Design review of the part built by this model. Coordinates are the model's own, in mm. A direction names the side the tool comes from. Give positions to 0.01 mm unless a question says otherwise; leave off trailing zeros. Order: outer loops, then holes, each group sorted by start corner. A loop starts at its lowest first (then second) coordinate and runs counter-clockwise, first axis right, second up.
```python
from build123d import *

# Parameters (mm, degrees)
BOSS_EXTRUDE1_DEPTH = 20
FILLET1_R           = 1
SKETCH2_R           = 9
CUT_EXTRUDE1_DEPTH  = 20
BOSS_EXTRUDE2_START = 2
BOSS_EXTRUDE2_DEPTH = 2
SKETCH4_W           = 20
SKETCH4_H           = 20
BOSS_EXTRUDE3_DEPTH = 2
FILLET2_R           = 1
SKETCH5_W           = 12.5
SKETCH5_H           = 2
CUT_EXTRUDE2_DEPTH  = 24
BOSS_EXTRUDE4_DEPTH = 80
FILLET3_R           = 1
SKETCH8_R           = 7.11392485
SKETCH8_W           = 20
SKETCH8_H           = 40
CUT_EXTRUDE3_DEPTH  = 2
SKETCH9_W           = 20
SKETCH9_H           = 2
BOSS_EXTRUDE5_DEPTH = 15
FILLET4_R           = 1
SKETCH10_R          = 2.5
CUT_EXTRUDE4_DEPTH  = 20
CUT_EXTRUDE5_DEPTH  = 1000
SKETCH12_W          = 38.052123651
SKETCH12_H          = 24.689337754
CUT_EXTRUDE6_DEPTH  = 200


with BuildPart() as part:
    # Sketch1 → Boss-Extrude1 (new body)
    with BuildSketch(Plane(origin=(0, 0, 0), x_dir=(1, 0, 0), z_dir=(0, 1, 0))):
        Polygon((-2.291666667, 11.041666667), (-22.291666667, 11.041666667), (-22.291666667, -8.958333333), (-2.291666667, -8.958333333), (-2.291666667, -6.958333333), (-20.291666667, -6.958333333), (-20.291666667, 9.041666667), (-2.291666667, 9.041666667), align=None)
    extrude(amount=BOSS_EXTRUDE1_DEPTH)

    # Fillet1
    fillet1_edges = [part.edges().sort_by_distance(p)[0] for p in [
        (-22.291666667, 10, 8.958333333),
        (-22.291666667, 10, -11.041666667),
    ]]
    fillet(fillet1_edges, radius=FILLET1_R)

    # Sketch2 → Cut-Extrude1 (cut)
    with BuildSketch(Plane.XY.offset(8.958333333)):
        with Locations(Location((-12.291666667, 10, 0), (0, 0, 180))):
            Circle(SKETCH2_R)
    extrude(amount=-CUT_EXTRUDE1_DEPTH, mode=Mode.SUBTRACT)

    # Sketch3 → Boss-Extrude2 (add)
    with BuildSketch(Plane(origin=(0, 20, 0), x_dir=(1, 0, 0), z_dir=(0, 1, 0)).offset(BOSS_EXTRUDE2_START)):
        Polygon((-2.291666667, 2.377848536), (-2.291666667, 9.041666667), (-20.291666667, 9.041666667), (-20.291666667, -6.958333333), (-2.291666667, -6.958333333), (-2.291666667, 0.377848536), align=None)
        with BuildLine():
            Line((-2.291666667, 9.041666667), (-2.291666667, 11.041666667))
            Line((-2.291666667, 11.041666667), (-21.291666667, 11.041666667))
            ThreePointArc((-21.291666667, 11.041666667), (-21.998773448, 10.748773448), (-22.291666667, 10.041666667))
            Line((-22.291666667, 10.041666667), (-22.291666667, -7.958333333))
            ThreePointArc((-22.291666667, -7.958333333), (-21.998773448, -8.665440115), (-21.291666667, -8.958333333))
            Line((-21.291666667, -8.958333333), (-2.291666667, -8.958333333))
            Line((-2.291666667, -8.958333333), (-2.291666667, -6.958333333))
            Line((-2.291666667, -6.958333333), (-20.291666667, -6.958333333))
            Line((-20.291666667, -6.958333333), (-20.291666667, 9.041666667))
            Line((-20.291666667, 9.041666667), (-2.291666667, 9.041666667))
        make_face()
    extrude(amount=-BOSS_EXTRUDE2_DEPTH)

    # Sketch4 → Boss-Extrude3 (add)
    with BuildSketch(Plane.XZ):
        with Locations((-12.291666667, -1.041666667)):
            Rectangle(SKETCH4_W, SKETCH4_H)
    extrude(amount=BOSS_EXTRUDE3_DEPTH)

    # Fillet2
    fillet2_edges = [part.edges().sort_by_distance(p)[0] for p in [
        (-22.291666667, -1, -11.041666667),
        (-22.291666667, -1, 8.958333333),
    ]]
    fillet(fillet2_edges, radius=FILLET2_R - 0.0001)  # a hair under: the kernel refuses the full size

    # Sketch5 → Cut-Extrude2 (cut)
    with BuildSketch(Plane(origin=(0, 22, 0), x_dir=(1, 0, 0), z_dir=(0, 1, 0))):
        with Locations((-8.541666667, 1.041666667)):
            Rectangle(SKETCH5_W, SKETCH5_H)
    extrude(amount=-CUT_EXTRUDE2_DEPTH, mode=Mode.SUBTRACT)

    # Sketch6 → Boss-Extrude4 (add)
    with BuildSketch(Plane.ZY.offset(22.291666667)):
        Polygon((2.408333333, -37), (0.408333333, -37), (0.408333333, -2), (0.408333333, 22), (2.408333333, 22), (2.408333333, -2), align=None)
    extrude(amount=BOSS_EXTRUDE4_DEPTH)

    # Fillet3
    fillet3_edges = [part.edges().sort_by_distance(p)[0] for p in [
        (-22.291666667, -37, 1.408333333),
        (-102.291666667, 22, 1.408333333),
        (-102.291666667, -37, 1.408333333),
    ]]
    fillet(fillet3_edges, radius=FILLET3_R)

    # Sketch8 → Cut-Extrude3 (cut)
    with BuildSketch(Plane(origin=(0, 0, 0.408333333), x_dir=(-1, 0, 0), z_dir=(0, 0, -1))):
        with Locations((12.291666667, 10)):
            Circle(SKETCH8_R)
        with Locations((82.291666667, -1)):
            Rectangle(SKETCH8_W, SKETCH8_H)
    extrude(amount=-CUT_EXTRUDE3_DEPTH, mode=Mode.SUBTRACT)

    # Sketch9 → Boss-Extrude5 (add, symmetric)
    with BuildSketch(Plane(origin=(0, 0, 0.408333333), x_dir=(-1, 0, 0), z_dir=(0, 0, -1))):
        Polygon((92.470978063, 20), (102.291666667, 20), (112.291666667, 20), (112.291666667, 18), (102.291666667, 18), (92.291666667, 18), (92.291666667, 20), align=None)
        with Locations((102.291666667, 1)):
            Rectangle(SKETCH9_W, SKETCH9_H)
    extrude(amount=BOSS_EXTRUDE5_DEPTH, both=True)

    # Fillet4
    fillet4_edges = [part.edges().sort_by_distance(p)[0] for p in [
        (-92.291666667, 19, 15.408333333),
        (-112.291666667, 19, 15.408333333),
        (-92.291666667, 19, -14.591666667),
        (-112.291666667, 19, -14.591666667),
        (-92.291666667, 1, 15.408333333),
        (-112.291666667, 1, 15.408333333),
        (-92.291666667, 1, -14.591666667),
        (-112.291666667, 1, -14.591666667),
    ]]
    fillet(fillet4_edges, radius=FILLET4_R)

    # Sketch10 → Cut-Extrude4 (cut)
    with BuildSketch(Plane.XZ):
        with Locations((-107.291666667, -1.848697286)):
            Circle(SKETCH10_R)
        with Locations((-107.291666667, -9.848697286)):
            Circle(SKETCH10_R)
    extrude(amount=-CUT_EXTRUDE4_DEPTH, mode=Mode.SUBTRACT)

    # Mirror1: part across plane


with BuildPart() as part_1:
    add(part.part)
    add(part.part.mirror(Plane.ZX.offset(22)))

    # Sketch11 → Cut-Extrude5 (cut)
    with BuildSketch(Plane.ZY.offset(102.291666667)):
        Polygon((0.408333333, 22), (17.6685399, 22), (17.6685399, -41.876309172), (-35.169754822, -41.876309172), (-35.169754822, 22), align=None)
    extrude(amount=-CUT_EXTRUDE5_DEPTH, mode=Mode.SUBTRACT)


with BuildPart() as cut_extrude5_piece_1:
    # of the separate pieces the step leaves, piece 1, a body of its own (cut_extrude5_pieces)
    add(part_1.part.solids().sort_by_distance((-101.291666667, 22, 2.408333333))[0])


with BuildPart() as cut_extrude5_piece_2:
    # of the separate pieces the step leaves, piece 2, a body of its own (cut_extrude5_pieces)
    add(part_1.part.solids().sort_by_distance((-102.291666667, 2, -14.591666667))[0])


with BuildPart() as cut_extrude5_piece_3:
    # of the separate pieces the step leaves, piece 3, a body of its own (cut_extrude5_pieces)
    add(part_1.part.solids().sort_by_distance((-111.291666667, 20, 15.408333333))[0])


with BuildPart() as cut_extrude6_tool:
    # Sketch12 → Cut-Extrude6 (new body)
    with BuildSketch(Plane.ZY.offset(112.291666667)):
        with Locations((0.662862589, 8.620210787)):
            Rectangle(SKETCH12_W, SKETCH12_H)
    extrude(amount=-CUT_EXTRUDE6_DEPTH)


with BuildPart() as cut_extrude5_piece_2_1:
    add(cut_extrude5_piece_2.part)

    # Cut-Extrude6: cut by cut_extrude6_tool
    add(cut_extrude6_tool.part, mode=Mode.SUBTRACT)


with BuildPart() as cut_extrude5_piece_3_1:
    add(cut_extrude5_piece_3.part)

    # Cut-Extrude6: cut by cut_extrude6_tool
    add(cut_extrude6_tool.part, mode=Mode.SUBTRACT)


solid = cut_extrude5_piece_1.part
```
1. Draft analysis for pull direction Z (two halves, no side actions). For faces 1 (the face through (-102, 44, 0)), 2 (the face through (-3, 31, 8.958)), 3 (the face through (-4, 30, -9.042)), state which applies: pulls with the +Z half, pulls with the -Z half, needs draft (parallel to the pull), parting line crosses it, or undercut.
Recorded:
face 1: needs draft
face 2: pulls with the +Z half
face 3: undercut
2. Take a section at B-B (y = 58.5). State the section outline as (x, z) points, then the cut area to 3 significant figures.
Recorded:
outline: (-102.29, 0.41) - (-92.29, 0.41) - (-92.29, 2.41) - (-102.29, 2.41) - close; (-72.29, 0.41) - (-22.29, 0.41) - (-22.29, 2.41) - (-72.29, 2.41) - close
area: 120 mm2
3. Take a section at A-A (x = -86). State the section outline as (y, z) points, then the cut area to 3 significant figures.
Recorded:
outline: (22, 0.41) - (25, 0.41) - (25, 2.41) - (22, 2.41) - close; (65, 0.41) - (81, 0.41) - (81, 2.41) - (65, 2.41) - close
area: 38.0 mm2
4. Machinability: for faces 4 (the face through (-14.792, 23, -1)), 5 (the face through (-3, 33, 6.958)), 6 (the face through (-92.292, 37, 1)), 7 (the face through (-102.292, 62, 1)), 8 (the face through (-3, 31, -11.042)), which of the approach directions +Z, -Z, +X, -X, +Y, -Y give a long, thin tool a straight path to every point of the face, cutting with its end or side? Answer none if there is none.
Recorded:
face 4: +X, +Y, -Y
face 5: +X
face 6: none
face 7: +Z, -Z, -X, +Y
face 8: -Z, +X, +Y, -Y
5. For line 1 along Y through (x, z) = (-95.5, -10.5); line 2 along X through (y, z) = (56, 2); line 3 along Z through (x, y) = (-42, 33), list the stretches that pass through material, from the lowest coordinate up.
Recorded:
line 1: y = 24 to 26, 42 to 44
line 2: x = -102.29 to -92.29, -72.29 to -22.29
line 3: z = 0.41 to 2.41
6. Take a section at D-D (x = -59.5). State the section outline as (y, z) points.
Recorded:
outline: (22, 0.41) - (81, 0.41) - (81, 2.41) - (22, 2.41) - close
7. For pin 1 (10 mm diameter, centred on y = 67.5, z = 5, fed in from -X); pin 2 (6.5 mm diameter, centred on x = -107.29, z = -9.85, fed in from -Y); pin 3 (8 mm diameter, centred on x = -97, y = 35, fed in from +Z), all flat-tipped, find the tip position at first contact; note any pin that passes through.
Recorded:
pin 1: stops at x = -102.29
pin 2: stops at y = 24
pin 3: stops at z = 2.41
8. Take a section at C-C (y = 71.5). State the section outline as (x, z) points.
Recorded:
outline: (-102.29, 0.41) - (-22.29, 0.41) - (-22.29, 2.41) - (-102.29, 2.41) - close
